Autodesk Inventor part; units mm, degrees
ref_plane "YZ Plane" through (0, 0, 0) normal (1, 0, 0) x (0, 1, 0)
ref_plane "XZ Plane" through (0, 0, 0) normal (0, 1, 0) x (-1, 0, 0)
ref_plane "XY Plane" through (0, 0, 0) normal (0, 0, 1) x (1, 0, 0)
sketch "Sketch1" plane through (0, 0, 0) normal (0, 0, 1) x (1, 0, 0)
  line L0 (-9.3, 0) -> (9.3, 0)
  line L1 (9.3, 0) -> (9.3, 5)
  line L2 (9.3, 5) -> (-9.3, 5)
  line L3 (-9.3, 5) -> (-9.3, 0)
  point P0 (0, 0)
  dimension "d2" = 18.6
  dimension "d3" = 9.3
  dimension "d4" = 5
  dimension "d7" = 0
extrude "Extrusion1" add sketch "Sketch1" along normal blind 3
sketch "Sketch2" plane through (0, 0, 3) normal (0, 0, 1) x (1, 0, 0)
  point P0 (0, 0)
sketch "Sketch3" plane through (0, 0, 3) normal (0, 0, 1) x (1, 0, 0)
  line L0 (9.3, 5) -> (-9.3, 5)
  line L1 (-9.3, 0) -> (9.3, 0)
  line L2 (-9.3, 5) -> (-5, 5)
  line L3 (-5, 5) -> (-5, 0)
  line L4 (-5, 0) -> (-9.3, 0)
  line L5 (-9.3, 0) -> (-9.3, 5)
  line L6 (0, 0) -> (0, 6.3784) construction
  line L7 (9.3, 5) -> (5, 5)
  line L8 (5, 5) -> (5, 0)
  line L9 (5, 0) -> (9.3, 0)
  line L10 (9.3, 0) -> (9.3, 5)
  point P0 (9.3, 0)
  dimension "d8" = 5
extrude "Extrusion2" add sketch "Sketch3" along normal blind 12.2 contours L10 L1 L8 L0 | L3 L1 L5 L0
sketch "Sketch4" plane through (0, 0, 0) normal (0, 0, -1) x (-1, 0, 0)
  line L0 (0, 1.1656) -> (-7.6, 1.1656) construction
  line L1 (0, 0) -> (0, 7.9667) construction
  line L2 (-8.0064, 1.6248) -> (-7.0594, 1.6248)
  line L3 (-7.0594, 1.6248) -> (-7.0594, 0.6778)
  line L4 (-7.0594, 0.6778) -> (-8.0064, 0.6778)
  line L5 (-8.0064, 0.6778) -> (-8.0064, 1.6248)
  line L6 (-9.3, 0) -> (-9.3, 5)
  line L7 (-9.3, 2.5) -> (9.3, 2.5) construction
  line L8 (9.3, 5) -> (9.3, 0)
  line L9 (-8.0064, 3.3752) -> (-7.0594, 3.3752)
  line L10 (-7.0594, 3.3752) -> (-7.0594, 4.3222)
  line L11 (-7.0594, 4.3222) -> (-8.0064, 4.3222)
  line L12 (-8.0064, 4.3222) -> (-8.0064, 3.3752)
  line L13 (8.0064, 1.6248) -> (7.0594, 1.6248)
  line L14 (7.0594, 1.6248) -> (7.0594, 0.6778)
  line L15 (7.0594, 0.6778) -> (8.0064, 0.6778)
  line L16 (8.0064, 0.6778) -> (8.0064, 1.6248)
  line L17 (8.0064, 3.3752) -> (7.0594, 3.3752)
  line L18 (7.0594, 3.3752) -> (7.0594, 4.3222)
  line L19 (7.0594, 4.3222) -> (8.0064, 4.3222)
  line L20 (8.0064, 4.3222) -> (8.0064, 3.3752)
  dimension "d11" = 7.6
extrude "Extrusion3" add sketch "Sketch4" along normal blind 12.2
properties part number "p_inter" material "PC/ABS Plastic"
Could you check a few things on this model? Use its own coordinates, in mm. A direction names the side the tool comes from. Round coordinates to 2 decimals unless told otherwise and drop trailing zeros. Write each loop counter-clockwise with the first axis right and the second up, starting at its lowest first coordinate (ties: lowest second). Pieces come first, ordered by that corner, then holes. Notation, with made-up numbers: M 8.25,39 L 52.25,39 A9 cw 52.25,45 Z; hole C 28,19.5 d3. An arc over 180 degrees is marked long. Answer in a Markdown table with one row per item. Add a question column.
Q1. Imagine slicing it at B-B (z = -8.5). Please give me the cut outline in (x, y).
Q2. If we mould it in two halves opening along Y, with no side actions, what happens to faces 1 (the flat face through (7.5, 1.625, -6)), 2 (the flat face through (7.5, 0.678, -6)), 3 (the flat face through (-7.5, 3.9, -12.2))? For each: +Y half, -Y half, draft (parallel to the pull), parting line (faces both ways), or undercut.
Q3. On a 3-axis mill with a long thin cutter (end or side, diameter ignored), from which of +Z, -Z, +X, -X, +Y, -Y can I reach the whole of each face in a straight line? I mean faces 4 (the flat face through (7.5, 3.375, -6)), 5 (the flat face through (-8.006, 4, -6)), 6 (the flat face through (7.5, 4.322, -6)), 7 (the flat face through (-7.059, 1, -6)). Say none if no direction works.
Q4. If I drill on line 1 (X direction, y = 0.9, z = -8.5); line 2 (X direction, y = 2.55, z = 12.25); line 3 (Y direction, x = 7.5, z = -6.75), over which ranges is the centre line in solid material (lowest first)? Write a range as from..to.
Q5. Imagine slicing it at D-D (x = -3.75). Please give me the cut outline in (y, z), then the cut area to 3 significant figures.
Q6. Imagine slicing it at C-C (y = 2.85). Please give me the cut outline in (x, z), then the cut area to 3 significant figures.
Q7. Will these pins go through, and if not, where does the flat tip stop? pin 1 Ø1.5 at (x, y) = (3.5, 3) entering from -Z; pin 2 Ø4 at (x, z) = (-4, 3.5) entering from +Y; pin 3 Ø2 at (x, y) = (-1, 0.5) entering from +Z; pin 4 Ø1 at (x, z) = (7.5, -7) entering from +Y.
Q8. Imagine slicing it at A-A (z = 11.5). Please give me the cut outline in (x, y), then the cut area to 3 significant figures.
Values:
| question | item | result |
|---|---|---|
| 1 | outline | M -8.01,0.68 L -7.06,0.68 L -7.06,1.62 L -8.01,1.62 Z; M -8.01,3.38 L -7.06,3.38 L -7.06,4.32 L -8.01,4.32 Z; M 7.06,0.68 L 8.01,0.68 L 8.01,1.62 L 7.06,1.62 Z; M 7.06,3.38 L 8.01,3.38 L 8.01,4.32 L 7.06,4.32 Z |
| 2 | face 1 | undercut |
| 2 | face 2 | -Y half |
| 2 | face 3 | draft |
| 3 | face 4 | -Z, +X, -X |
| 3 | face 5 | -Z, -X, +Y, -Y |
| 3 | face 6 | -Z, +X, -X, +Y |
| 3 | face 7 | -Z, +Y, -Y |
| 4 | line 1 | -8.01..-7.06, 7.06..8.01 |
| 4 | line 2 | -9.3..-5, 5..9.3 |
| 4 | line 3 | 0.68..1.62, 3.38..4.32 |
| 5 | outline | M 0,0 L 5,0 L 5,3 L 0,3 Z |
| 5 | area | 15.0 mm^2 |
| 6 | outline | M -9.3,0 L 9.3,0 L 9.3,15.2 L 5,15.2 L 5,3 L -5,3 L -5,15.2 L -9.3,15.2 Z |
| 6 | area | 161 mm^2 |
| 7 | pin 1 | z = 0 |
| 7 | pin 2 | y = 5 |
| 7 | pin 3 | z = 3 |
| 7 | pin 4 | y = 4.32 |
| 8 | outline | M -9.3,0 L -5,0 L -5,5 L -9.3,5 Z; M 5,0 L 9.3,0 L 9.3,5 L 5,5 Z |
| 8 | area | 43.0 mm^2 |
